The listing builds one solid part. Answer for the finished solid, in the listing's coordinates (mm). A direction names the side the tool comes from. Give positions to 0.01 mm unless a question says otherwise; leave off trailing zeros. Loops run counter-clockwise (first coordinate to the right, second up) from the corner with the lowest first, then second, coordinate; pieces in that order, holes last. Notation, with made-up numbers: (4, 37.25) - (13, 37.25) arc R7 cw to (13, 41.25) - close; hole circle Ø6 at (-25, 12). An arc over 180 degrees is marked (long way). One line per item, written item: value. Start each with the question number.
from build123d import *

# Parameters (mm, degrees)
SKETCH2_R           = 6
BOSS_EXTRUDE1_DEPTH = 2
CUT_EXTRUDE3_DEPTH  = 4


with BuildPart() as part:
    # Sketch2 → Boss-Extrude1 (new body)
    with BuildSketch(Plane(origin=(0, 0, 0), x_dir=(1, 0, 0), z_dir=(0, 1, 0))):
        with Locations(Location((0, 0, 0), (0, 0, 270))):
            Circle(SKETCH2_R)
    extrude(amount=BOSS_EXTRUDE1_DEPTH)

    # Sketch3 → Cut-Extrude3 (cut)
    with BuildSketch(Plane(origin=(0, 2, 0), x_dir=(1, 0, 0), z_dir=(0, 1, 0))):
        with BuildLine():
            Line((-2.179449472, 0.3), (0, 0.3))
            Line((0, 0.3), (2.179449472, 0.3))
            ThreePointArc((2.179449472, 0.3), (0, 2.2), (-2.179449472, 0.3))
        make_face()
        with BuildLine():
            Line((2.179449472, -0.3), (0, -0.3))
            Line((0, -0.3), (-2.179449472, -0.3))
            ThreePointArc((-2.179449472, -0.3), (0, -2.2), (2.179449472, -0.3))
        make_face()
    extrude(amount=-CUT_EXTRUDE3_DEPTH, mode=Mode.SUBTRACT)


solid = part.part
1. A cutting plane is placed at B-B (y = 0.35). Determine the outline of the cut face in (x, z), plus the area to 3 significant figures.
2. Flat-ended cylindrical pins translate along their axes: pin 1 (0.6 mm diameter, centred on x = 0.5, y = 0.5, fed in from -Z); pin 2 (1 mm diameter, centred on x = 1.5, z = -1, fed in from -Y); pin 3 (1 mm diameter, centred on x = -1, y = 1, fed in from +Z). Find the tip coordinate at first contact, or state that the pin passes through.
3. A cutting plane is placed at A-A (x = 0). Determine the outline of the cut face in (y, z).
4. A cutting plane is placed at D-D (z = 3.75). Determine the outline of the cut face in (x, y), plus the area to 3 significant figures.
5. Find the intervals of material crossed by L1, parallel to Z at x = -1, y = 1.8; L2, parallel to Z at x = 0.75, y = 1.4; L3, parallel to X at y = 1.2, z = 0.75, in increasing order. Write a range as [from, to].
6. A cutting plane is placed at C-C (x = 2). Determine the outline of the cut face in (y, z), plus the area to 3 significant figures.
7. For faces 4 (the flat face through (0, 1, 0.3)), 5 (the flat face through (0, 0, 0)), determine the directions among +Z, -Z, +X, -X, +Y, -Y from which every point of the face is accessible in a straight line to the end or side of a thin tool.
8. Determine the mould class of faces 1 (the flat face through (0, 1, -0.3)), 2 (the cylindrical face through (1.802, 0.986, 5.723)), 3 (the flat face through (0, 2, 0)) for opening direction Z: released by +Z, released by -Z, zero draft, split by the parting line, or undercut.
Results below:
1. outline: circle Ø12 at (0, 0); hole (-2.18, -0.3) arc R2.2 ccw to (2.18, -0.3) - close; hole (-2.18, 0.3) - (2.18, 0.3) arc R2.2 ccw to start
1. area: 101 mm^2
2. pin 1: stops at z = -6
2. pin 2: stops at y = 0
2. pin 3: stops at z = 5.98
3. outline: (0, -6) - (2, -6) - (2, -2.2) - (0, -2.2) - close; (0, -0.3) - (2, -0.3) - (2, 0.3) - (0, 0.3) - close; (0, 2.2) - (2, 2.2) - (2, 6) - (0, 6) - close
4. outline: (-4.68, 0) - (4.68, 0) - (4.68, 2) - (-4.68, 2) - close
4. area: 18.7 mm^2
5. L1: z = [-5.92, -1.96], [-0.3, 0.3], [1.96, 5.92]
5. L2: z = [-5.95, -2.07], [-0.3, 0.3], [2.07, 5.95]
5. L3: x = [-5.95, -2.07], [2.07, 5.95]
6. outline: (0, -5.66) - (2, -5.66) - (2, -0.92) - (0, -0.92) - close; (0, -0.3) - (2, -0.3) - (2, 0.3) - (0, 0.3) - close; (0, 0.92) - (2, 0.92) - (2, 5.66) - (0, 5.66) - close
6. area: 20.2 mm^2
7. face 4: +Y, -Y
7. face 5: +Z, -Z, +X, -X, -Y
8. face 1: undercut
8. face 2: split by the parting line
8. face 3: zero draft
